```python
from build123d import *

# Parameters (mm, degrees)
SKETCH1_W           = 205
SKETCH1_H           = 166.5
BOSS_EXTRUDE1_DEPTH = 20
CUT_EXTRUDE1_DEPTH  = 2
CUT_EXTRUDE3_DEPTH  = 38


with BuildPart() as part:
    # Sketch1 → Boss-Extrude1 (new, symmetric)
    with BuildSketch(Plane(origin=(0, 0, 0), x_dir=(1, 0, 0), z_dir=(0, 1, 0))):
        Rectangle(SKETCH1_W, SKETCH1_H)
    extrude(amount=BOSS_EXTRUDE1_DEPTH, both=True)

    # Sketch3 → Cut-Extrude1 (cut)
    # profile 1 of 4: a face of its own
    with BuildSketch(Plane(origin=(0, 20, 0), x_dir=(1, 0, 0), z_dir=(0, 1, 0))):
        Polygon((-100.5, -81.25), (-100.5, 5.75), (-100.5, 81.25), (-7, 81.25), (-7, 75.25), (-94.5, 75.25), (-94.5, 13.75), (-37, 13.75), (-37, 5.75), (-37, 2.25), (-96.5, 2.25), (-96.5, -77.25), (96.5, -77.25), (96.5, 2.25), (37, 2.25), (37, 5.75), (37, 13.75), (94.5, 13.75), (94.5, 75.25), (7, 75.25), (7, 81.25), (100.5, 81.25), (100.5, 5.75), (100.5, -81.25), align=None)
        Polygon((7.5, 80.75), (100, 80.75), (100, 5.75), (100, -80.75), (-100, -80.75), (-100, 5.75), (-100, 80.75), (-7.5, 80.75), (-7.5, 75.75), (-95, 75.75), (-95, 13.25), (-37.5, 13.25), (-37.5, 5.75), (-37.5, 2.75), (-97, 2.75), (-97, -77.75), (97, -77.75), (97, 2.75), (37.5, 2.75), (37.5, 5.75), (37.5, 13.25), (95, 13.25), (95, 75.75), (7.5, 75.75), align=None, mode=Mode.SUBTRACT)
    # profile 2 of 4: a face of its own
    with BuildSketch(Plane(origin=(0, 20, 0), x_dir=(1, 0, 0), z_dir=(0, 1, 0))):
        Polygon((-100, -80.75), (-100, 5.75), (-37.5, 5.75), (-37.5, 2.75), (-97, 2.75), (-97, -77.75), (97, -77.75), (97, 2.75), (37.5, 2.75), (37.5, 5.75), (100, 5.75), (100, -80.75), align=None)
    # profile 3 of 4: a face of its own
    with BuildSketch(Plane(origin=(0, 20, 0), x_dir=(1, 0, 0), z_dir=(0, 1, 0))):
        Polygon((-95, 13.25), (-37.5, 13.25), (-37.5, 5.75), (-100, 5.75), (-100, 80.75), (-7.5, 80.75), (-7.5, 75.75), (-95, 75.75), align=None)
    # profile 4 of 4: a face of its own
    with BuildSketch(Plane(origin=(0, 20, 0), x_dir=(1, 0, 0), z_dir=(0, 1, 0))):
        Polygon((100, 80.75), (100, 5.75), (37.5, 5.75), (37.5, 13.25), (95, 13.25), (95, 75.75), (7.5, 75.75), (7.5, 80.75), align=None)
    extrude(amount=-CUT_EXTRUDE1_DEPTH, mode=Mode.SUBTRACT)

    # Sketch5 → Cut-Extrude3 (cut)
    with BuildSketch(Plane(origin=(0, 20, 0), x_dir=(1, 0, 0), z_dir=(0, 1, 0))):
        Polygon((-7, 73.75), (7, 73.75), (93, 73.75), (93, 15.25), (35.5, 15.25), (35.5, 0.75), (95, 0.75), (95, -75.75), (-95, -75.75), (-95, 0.75), (-35.5, 0.75), (-35.5, 15.25), (-93, 15.25), (-93, 73.75), align=None)
    extrude(amount=-CUT_EXTRUDE3_DEPTH, mode=Mode.SUBTRACT)


solid = part.part
```
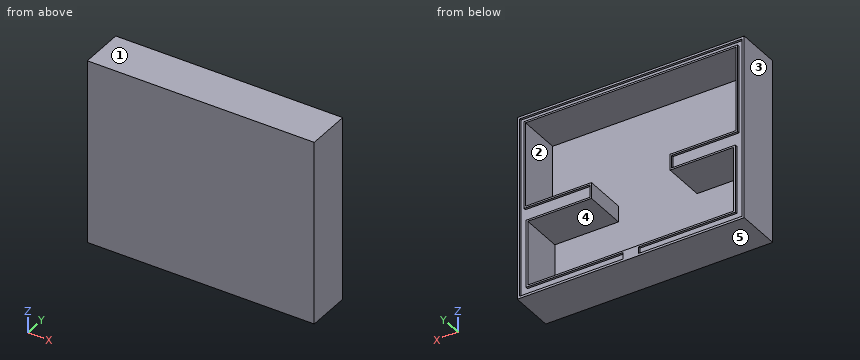
Work out the finished part from the listing and answer in its coordinate system (mm). Face numbers are marked on the shaded views. A direction names the side the tool comes from. Give positions to 0.01 mm unless a question says otherwise; leave off trailing zeros. Loops run counter-clockwise (first coordinate to the right, second up) from the corner with the lowest first, then second, coordinate; pieces in that order, holes last. Notation, with made-up numbers: (-21.75, 17) -> (21.25, 17) arc R22 cw to (21.25, 38) -> close; hole circle Ø1 at (39.5, 80.25). An arc over 180 degrees is marked (long way). Put each result on its own line as item: value. Start each with the question number.
Item 1: The part is cut by section B-B (x = 9.5). Give the vertices of the cut face in (y, z).
Item 2: The part is cut by section D-D (x = 75.5). Give the vertices of the cut face in (y, z).
Item 3: Find the intervals of material crossed by L1, parallel to Z at x = 78, y = -5.5; L2, parallel to X at y = -12, z = 11.5; L3, parallel to Z at x = 14.5, y = -7, in increasing order. Write a range as [from, to].
Item 4: The part is cut by section C-C (z = -55). Give the vertices of the cut face in (x, y), then the cut area to 3 significant figures.
Item 5: The mould has two halves that part along Z. Classify the marked faces 1, 2 and 3: released by +Z, released by -Z, zero draft, split by the parting line, or undercut.
Item 6: The part is cut by section A-A (y = 0). Give the vertices of the cut face in (x, z), then the cut area to 3 significant figures.
Item 7: Which of the six approach directions +Z, -Z, +X, -X, +Y, -Y give full straight-line access (tool end or side, diameter ignored) to the marked faces 4 and 5?
Answers below:
1. outline: (-20, -83.25) -> (20, -83.25) -> (20, -81.25) -> (18, -81.25) -> (18, -75.25) -> (20, -75.25) -> (20, -73.75) -> (-18, -73.75) -> (-18, 75.75) -> (20, 75.75) -> (20, 77.25) -> (18, 77.25) -> (18, 81.25) -> (20, 81.25) -> (20, 83.25) -> (-20, 83.25) -> close
2. outline: (-20, -83.25) -> (20, -83.25) -> (20, -81.25) -> (18, -81.25) -> (18, -75.25) -> (20, -75.25) -> (20, -73.75) -> (-18, -73.75) -> (-18, -15.25) -> (20, -15.25) -> (20, -13.75) -> (18, -13.75) -> (18, -2.25) -> (20, -2.25) -> (20, -0.75) -> (-18, -0.75) -> (-18, 75.75) -> (20, 75.75) -> (20, 77.25) -> (18, 77.25) -> (18, 81.25) -> (20, 81.25) -> (20, 83.25) -> (-20, 83.25) -> close
3. L1: [-83.25, -73.75], [-15.25, -0.75], [75.75, 83.25]
3. L2: [-102.5, -95], [95, 102.5]
3. L3: [-83.25, -73.75], [75.75, 83.25]
4. outline: (-102.5, -20) -> (102.5, -20) -> (102.5, 20) -> (100.5, 20) -> (100.5, 18) -> (94.5, 18) -> (94.5, 20) -> (93, 20) -> (93, -18) -> (-93, -18) -> (-93, 20) -> (-94.5, 20) -> (-94.5, 18) -> (-100.5, 18) -> (-100.5, 20) -> (-102.5, 20) -> close
4. area: 1,110 mm2
5. face 1: released by +Z
5. face 2: undercut
5. face 3: zero draft
6. outline: (-102.5, -83.25) -> (102.5, -83.25) -> (102.5, 83.25) -> (-102.5, 83.25) -> close; hole (-95, -0.75) -> (-35.5, -0.75) -> (-35.5, -15.25) -> (-93, -15.25) -> (-93, -73.75) -> (93, -73.75) -> (93, -15.25) -> (35.5, -15.25) -> (35.5, -0.75) -> (95, -0.75) -> (95, 75.75) -> (-95, 75.75) -> close
6. area: 7,690 mm2
7. face 4: +Y
7. face 5: -Z, +X, -X, +Y, -Y
